Source: CAD feature listing. Evaluate the final solid. Frame: model axes, mm. A direction names the side the tool comes from. Give positions to 0.01 mm unless a question says otherwise; leave off trailing zeros. Order: outer loops, then holes, each group sorted by start corner. A loop starts at its lowest first (then second) coordinate and runs counter-clockwise, first axis right, second up. Notation, with made-up numbers: M 51,13 L 108,13 A19 ccw 108,29 Z; hole C 72.25,-5.75 d7. An arc over 180 degrees is marked long. Answer in a Markdown table with one row per item. Add a question column.
(1) Material intervals for line 1 along Y through (x, z) = (64.45, -2.5); line 2 along X through (y, z) = (52.5, -4.5); line 3 along Y through (x, z) = (62, 1.5), sorted ascending.
(2) Set-up query: faces 1 (the face through (63, 66, 1)), 2 (the face through (1, 29.5, -2)), 3 (the face through (2, 52, -2)), 4 (the face through (64, 27, -2)), 5 (the face through (64, 52, -2)). Return all of +Z, -Z, +X, -X, +Y, -Y with unobstructed straight access to the full face (end or side cutting, diameter ignored); none if empty.
(3) Mould query, pull axis X, two halves, no side actions, for faces 6 (the face through (58, 61, 1)), 7 (the face through (65, 29.5, -2)), 8 (the face through (66, 39, -0.8)). Classes: pulls with the +X half, pulls with the -X half, needs draft (parallel to the pull), parting line crosses it, or undercut.
(4) Section query A-A, the plane y = 69. Return loops of the section in (x, z), plus the area to 3 significant figures.
(5) Section query D-D, the plane y = 39.5. Return loops of the section in (x, z), plus the area to 3 significant figures.
(6) Pin query (flat end, axial travel): P1, Ø1, axis at x = 65.5, z = -3.5, coming from the +Y side; P2, Ø0.6, axis at x = 65.5, z = -3, coming from the -Y side; P3, Ø3, axis at x = 56, z = -3, coming from the +Y side; P4, Ø1.1, axis at x = 2.5, z = -3.5, coming from the -Y side. Return the tip coordinate at first contact, or that it passes through.
(7) Section query B-B, the plane z = -2.5. Return loops of the section in (x, y).
(8) Section query C-C, the plane x = 57.5. Return loops of the section in (y, z), plus the area to 3 significant figures.
from build123d import *

# Parameters (mm, degrees)
BOX_W                  = 66
BOX_H                  = 79
BOX_DEPTH              = 2
FILLET_R               = 2
BOX001_W               = 10
BOX001_H               = 10
BOX001_DEPTH           = 2
FILLET001_R            = 1
BOX002_W               = 2
BOX002_H               = 20
BOX002_DEPTH           = 5
LINEARPATTERN_COUNT    = 2
LINEARPATTERN_PITCH    = 64
BOX003_W               = 1
BOX003_H               = 30
BOX003_DEPTH           = 5
LINEARPATTERN001_COUNT = 2
LINEARPATTERN001_PITCH = 61
CYLINDER_R             = 1.5
CYLINDER_DEPTH         = 3
LINEARPATTERN002_COUNT = 2
LINEARPATTERN002_PITCH = 63


with BuildPart() as part:
    # Box → Box (join)
    with BuildSketch(Plane.XY):
        with Locations((33, 39.5)):
            Rectangle(BOX_W, BOX_H)
    extrude(amount=BOX_DEPTH)

    # Fillet
    fillet_edges = [part.edges().sort_by_distance(p)[0] for p in [
        (0, 0, 1),
        (66, 0, 1),
        (66, 79, 1),
        (0, 79, 1),
    ]]
    fillet(fillet_edges, radius=FILLET_R)

    # Box001 → Box001 (cut)
    with BuildSketch(Plane(origin=(53, 61, 0), x_dir=(1, 0, 0), z_dir=(0, 0, 1))):
        with Locations((5, 5)):
            Rectangle(BOX001_W, BOX001_H)
    extrude(amount=BOX001_DEPTH, mode=Mode.SUBTRACT)

    # Fillet001
    fillet001_edges = [part.edges().sort_by_distance(p)[0] for p in [
        (53, 71, 1),
        (63, 71, 1),
        (53, 61, 1),
        (63, 61, 1),
    ]]
    fillet(fillet001_edges, radius=FILLET001_R)

    # Box002 → Box002 (join)
    with BuildSketch(Plane(origin=(64, 49.5, 0), x_dir=(1, 0, 0), z_dir=(0, 0, -1))):
        with Locations((1, 10)):
            Rectangle(BOX002_W, BOX002_H)
    box002 = extrude(amount=BOX002_DEPTH)

    # LinearPattern: Box002 ×2
    with Locations(*[(-i * LINEARPATTERN_PITCH, 0, 0) for i in range(1, LINEARPATTERN_COUNT)]):
        add(box002)

    # Box003 → Box003 (join)
    with BuildSketch(Plane(origin=(63, 54.5, 0), x_dir=(1, 0, 0), z_dir=(0, 0, -1))):
        with Locations((0.5, 15)):
            Rectangle(BOX003_W, BOX003_H)
    box003 = extrude(amount=BOX003_DEPTH)

    # LinearPattern001: Box003 ×2
    with Locations(*[(-i * LINEARPATTERN001_PITCH, 0, 0) for i in range(1, LINEARPATTERN001_COUNT)]):
        add(box003)

    # Cylinder → Cylinder (cut)
    with BuildSketch(Plane(origin=(63, 39.5, -2.5), x_dir=(0, -1, 0), z_dir=(1, 0, 0))):
        Circle(CYLINDER_R)
    cylinder = extrude(amount=CYLINDER_DEPTH, mode=Mode.SUBTRACT)

    # LinearPattern002: Cylinder ×2
    with Locations(*[(-i * LINEARPATTERN002_PITCH, 0, 0) for i in range(1, LINEARPATTERN002_COUNT)]):
        add(cylinder, mode=Mode.SUBTRACT)


solid = part.part
Values follow:
| question | item | result |
|---|---|---|
| 1 | line 1 | y = 29.5 to 38, 41 to 49.5 |
| 1 | line 2 | x = 2 to 3, 63 to 64 |
| 1 | line 3 | y = 0 to 61, 71 to 79 |
| 2 | face 1 | +Z, -Z |
| 2 | face 2 | -Z, -X, -Y |
| 2 | face 3 | -Z, -X, +Y |
| 2 | face 4 | -Z, +X, -Y |
| 2 | face 5 | -Z, +X, +Y |
| 3 | face 6 | undercut |
| 3 | face 7 | needs draft |
| 3 | face 8 | pulls with the +X half |
| 4 | outline | M 0,0 L 53,0 L 53,2 L 0,2 Z; M 63,0 L 66,0 L 66,2 L 63,2 Z |
| 4 | area | 112 mm² |
| 5 | outline | M 0,-5 L 3,-5 L 3,-4 L 0,-4 Z; M 0,-1 L 3,-1 L 3,0 L 63,0 L 63,-1 L 66,-1 L 66,2 L 0,2 Z; M 63,-5 L 66,-5 L 66,-4 L 63,-4 Z |
| 5 | area | 144 mm² |
| 6 | P1 | stops at y = 49.5 |
| 6 | P2 | stops at y = 29.5 |
| 6 | P3 | passes through |
| 6 | P4 | stops at y = 24.5 |
| 7 | outline | M 0,29.5 L 2,29.5 L 2,24.5 L 3,24.5 L 3,38 L 0,38 Z; M 0,41 L 3,41 L 3,54.5 L 2,54.5 L 2,49.5 L 0,49.5 Z; M 63,24.5 L 64,24.5 L 64,29.5 L 66,29.5 L 66,38 L 63,38 Z; M 63,41 L 66,41 L 66,49.5 L 64,49.5 L 64,54.5 L 63,54.5 Z |
| 8 | outline | M 0,0 L 61,0 L 61,2 L 0,2 Z; M 71,0 L 79,0 L 79,2 L 71,2 Z |
| 8 | area | 138 mm² |
